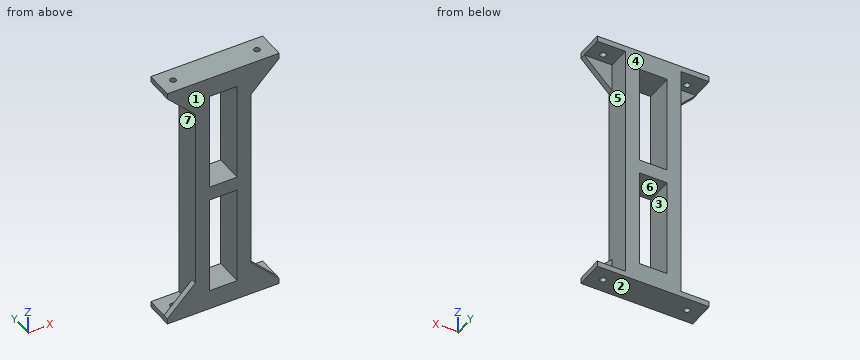
```python
from build123d import *

# Parameters (mm, degrees)
BOSS_EXTRUDE1_DEPTH = 20
BOSS_EXTRUDE2_DEPTH = 4
SKETCH3_W           = 20
SKETCH3_H           = 71
CUT_EXTRUDE1_DEPTH  = 55
SKETCH6_R           = 2.1
CUT_EXTRUDE2_DEPTH  = 207


with BuildPart() as part:
    # Sketch1 → Boss-Extrude1 (new body)
    with BuildSketch(Plane(origin=(0, 0, 0), x_dir=(1, 0, 0), z_dir=(0, 1, 0))):
        Polygon((20, 176), (20, 4), (0, 4), (0, 0), (80, 0), (80, 4), (60, 4), (60, 176), (80, 176), (80, 180), (0, 180), (0, 176), align=None)
    extrude(amount=BOSS_EXTRUDE1_DEPTH)

    # Sketch2 → Boss-Extrude2 (add)
    with BuildSketch(Plane.XZ):
        Polygon((60, -4), (60, -24), (80, -4), align=None)
        Polygon((0, -4), (20, -24), (20, -4), align=None)
        Polygon((0, -176), (20, -176), (20, -156), align=None)
        Polygon((60, -176), (80, -176), (60, -156), align=None)
    extrude(amount=-BOSS_EXTRUDE2_DEPTH)

    # Sketch3 → Cut-Extrude1 (cut)
    with BuildSketch(Plane(origin=(0, 20, 0), x_dir=(1, 0, 0), z_dir=(0, 1, 0))):
        with Locations((40, 49.5)):
            Rectangle(SKETCH3_W, SKETCH3_H)
        with Locations((40, 130.5)):
            Rectangle(SKETCH3_W, SKETCH3_H)
    extrude(amount=-CUT_EXTRUDE1_DEPTH, mode=Mode.SUBTRACT)

    # Sketch6 → Cut-Extrude2 (cut)
    with BuildSketch(Plane.XY):
        with Locations((10, 10)):
            Circle(SKETCH6_R)
        with Locations((70, 10)):
            Circle(SKETCH6_R)
    extrude(amount=-CUT_EXTRUDE2_DEPTH, mode=Mode.SUBTRACT)


solid = part.part
```
Geometry: final body of the model. Coordinates: model frame, mm. Face numbers are marked on the shaded views. A direction names the side the tool comes from. Round coordinates to 2 decimals unless told otherwise and drop trailing zeros. Order: outer loops, then holes, each group sorted by start corner. A loop starts at its lowest first (then second) coordinate and runs counter-clockwise, first axis right, second up. Notation, with made-up numbers: (85.5, 27.5) -> (132.5, 27.5) arc R12 ccw to (132.5, 39.5) -> close; hole circle Ø4 at (3.25, 23.25). An arc over 180 degrees is marked (long way). Use one line per item in the form item = value.
(1) First-contact query: pin 1 Ø5 at (y, z) = (13, -117.5) entering from -X; pin 2 Ø3.5 at (x, y) = (10, 10) entering from +Z; pin 3 Ø1.5 at (y, z) = (3.5, -40.5) entering from +X; pin 4 Ø10 at (y, z) = (3, -26.5) entering from +X. Flat tips, straight axial feed; report the tip coordinate or a pass-through.
Results list:
pin_1 = 20
pin_2 = through
pin_3 = 60
pin_4 = 62.5
(2) Section C-C on x = 37. Return loops of the section in (y, z).
Results list:
outline = (0, -180) -> (20, -180) -> (20, -166) -> (0, -166) -> close; (0, -95) -> (20, -95) -> (20, -85) -> (0, -85) -> close; (0, -14) -> (20, -14) -> (20, 0) -> (0, 0) -> close
(3) Draft query along Z for the marked faces 1, 2 and 3. Return one class per face: pulls with the +Z half, pulls with the -Z half, needs draft (parallel to the pull), parting line crosses it, or undercut.
Results list:
face_1 = needs draft
face_2 = pulls with the -Z half
face_3 = undercut
(4) Access query for the marked faces 4, 5, 6 and 7. Directions: +Z, -Z, +X, -X, +Y, -Y. A direction counts if a zero-diameter tool reaches every point of the face in a straight line with its end or side. Return the directions, or none.
Results list:
face_4 = +Z, -Z, +X, -X, +Y
face_5 = +X, +Y
face_6 = +Y, -Y
face_7 = -X, +Y
(5) Section A-A on x = 5.5. Return loops of the section in (y, z), and give its area (3 significant figures).
Results list:
outline = (0, -180) -> (20, -180) -> (20, -176) -> (4, -176) -> (4, -170.5) -> (0, -170.5) -> close; (0, -9.5) -> (4, -9.5) -> (4, -4) -> (20, -4) -> (20, 0) -> (0, 0) -> close
area = 204 mm^2
(6) Ray query, probe 1 along Z at (x, y) = (41.5, 4); probe 2 along X at (y, z) = (6, -117); probe 3 along Z at (x, y) = (63, 17.5). Return the intervals inside material, ascending. Write a range as [from, to].
Results list:
probe_1 = [-180, -166], [-95, -85], [-14, 0]
probe_2 = [20, 30], [50, 60]
probe_3 = [-180, -176], [-4, 0]
(7) Section B-B on z = -126. Return loops of the section in (x, y).
Results list:
outline = (20, 0) -> (30, 0) -> (30, 20) -> (20, 20) -> close; (50, 0) -> (60, 0) -> (60, 20) -> (50, 20) -> close
(8) Section D-D on y = 10. Count the separate pieces of the cut face and the enclosed holes in it, and give its area (3 significant figures).
Results list:
separate_pieces = 5
enclosed_holes = 2
area = 4,610 mm^2
